Can you work these out from the model? Positions are in its coordinate system, mm. A direction names the side the tool comes from. Give positions to 0.01 mm unless a question says otherwise; leave off trailing zeros. Order: outer loops, then holes, each group sorted by start corner. A loop starts at its lowest first (then second) coordinate and runs counter-clockwise, first axis right, second up. Notation, with made-up numbers: (-2.75, 69.25) - (33.25, 69.25) arc R26 ccw to (33.25, 96.25) - close; hole circle Ø8 at (10, 5.5). An arc over 180 degrees is marked (long way). Answer as a JSON object with one key per item and string values.
Autodesk Inventor part; units mm, degrees
ref_plane "YZ Plane" through (0, 0, 0) normal (1, 0, 0) x (0, 1, 0)
ref_plane "XZ Plane" through (0, 0, 0) normal (0, 1, 0) x (-1, 0, 0)
ref_plane "XY Plane" through (0, 0, 0) normal (0, 0, 1) x (1, 0, 0)
sketch "Sketch1" plane through (0, 0, 0) normal (0, 0, 1) x (1, 0, 0)
  circle A0 centre (0, 0) radius 32
  circle A1 centre (20, 0) radius 2.5
  circle A2 centre (-10, 17.3205) radius 2.5
  circle A3 centre (-10, -17.3205) radius 2.5
  dimension "d0" = 64
  dimension "d1" = 5
  dimension "d2" = 20
  dimension "d5" = 360
extrude "Extrusion1" add sketch "Sketch1" along normal blind 15
sketch "Sketch2" plane through (0, 0, 0) normal (0, 0, -1) x (-1, 0, 0)
  circle A0 centre (0, 0) radius 4.5
  dimension "d9" = 9
extrude "Extrusion2" cut sketch "Sketch2" against normal blind 5
fillet "Fillet1" radius 8 1 edges at (-32, 0, 15)
properties part number "AA013" material "ABS Plastic"
Q1. If we section it at C-C, the plane z = 7.75: Please give me the cut outline in (x, y), then the cut area to 3 significant figures.
Recorded:
{"outline": "circle Ø63.93 at (0, 0); hole circle Ø5 at (-10, -17.32); hole circle Ø5 at (-10, 17.32); hole circle Ø5 at (20, 0)", "area": "3,150 mm^2"}
Q2. If we section it at A-A, the plane y = 0: Please give me the cut outline in (x, z).
Recorded:
{"outline": "(-32, 0) - (-4.5, 0) - (-4.5, 5) - (4.5, 5) - (4.5, 0) - (17.5, 0) - (17.5, 15) - (-24, 15) arc R8 ccw to (-32, 7) - close; (22.5, 0) - (32, 0) - (32, 7) arc R8 ccw to (24, 15) - (22.5, 15) - close"}
Q3. If we section it at D-D, the plane x = -10: Count the separate pieces of the cut face and the enclosed holes in it, then the cut area to 3 significant figures.
Recorded:
{"separate pieces": "3", "enclosed holes": "0", "area": "733 mm^2"}
Q4. I need wall thicknesses on L1, parallel to Y at x = 0, z = 3.05; L2, parallel to X at y = -0.5, z = 3; L3, parallel to Y at x = -11, z = 9. Which ranges of each line are inside material? Lowest first, please.
Recorded:
{"L1": "y = -32 to -4.5, 4.5 to 32", "L2": "x = -32 to -4.47, 4.47 to 17.55, 22.45 to 32", "L3": "y = -29.78 to -19.61, -15.03 to 15.03, 19.61 to 29.78"}
Q5. If we section it at B-B, the plane x = 0: Please give me the cut outline in (y, z).
Recorded:
{"outline": "(-32, 0) - (-4.5, 0) - (-4.5, 5) - (4.5, 5) - (4.5, 0) - (32, 0) - (32, 7) arc R8 ccw to (24, 15) - (-24, 15) arc R8 ccw to (-32, 7) - close"}
Q6. Which directions (+Z, -Z, +X, -X, +Y, -Y) give clear straight access to the entire face, cutting with the end or side of a thin tool? Please do faces 1 (the face through (0, 0, 15)), 2 (the face through (0.59, 4.46, 2.46)).
Recorded:
{"face 1": "+Z, +X, -X, +Y, -Y", "face 2": "-Z"}
Q7. I'm going to push flat-ended pins straight in: pin 1 Ø2.5 at (x, y) = (-2, 0) entering from -Z; pin 2 Ø1.5 at (x, z) = (20, 10.5) entering from +Y; pin 3 Ø8 at (x, z) = (-5, 13) entering from -Y. Where does each tip first touch, or does it pass through?
Recorded:
{"pin 1": "stops at z = 5", "pin 2": "stops at y = 24.69", "pin 3": "stops at y = -31.47"}
Q8. We'd pull the mould along X, two halves only. Please class faces 3 (the face through (-6.94, 31.24, 3.45)), 4 (the face through (0, -7, 0)), 5 (the face through (-10.54, 19.76, 7.4)): released by +X, released by -X, zero draft, split by the parting line, or undercut.
Recorded:
{"face 3": "split by the parting line", "face 4": "zero draft", "face 5": "undercut"}
